Input: part model. Units: mm. Frame: model coordinates. A direction names the side the tool comes from. Coordinates: 2 decimals unless noted, no trailing zeros. Order: outer loops, then holes, each group sorted by start corner. A loop starts at its lowest first (then second) coordinate and runs counter-clockwise, first axis right, second up. Notation, with made-up numbers: (46.5, 18.5) -> (87.5, 18.5) arc R29 ccw to (87.5, 49.5) -> close; hole circle Ø10 at (50, 0.25). An arc over 180 degrees is marked (long way). Write each question's results on one line, items separated by ' | '.
Autodesk Inventor part; units mm, degrees
ref_plane "YZ Plane" through (0, 0, 0) normal (1, 0, 0) x (0, 1, 0)
ref_plane "XZ Plane" through (0, 0, 0) normal (0, 1, 0) x (-1, 0, 0)
ref_plane "XY Plane" through (0, 0, 0) normal (0, 0, 1) x (1, 0, 0)
sketch "Schizzo1" plane through (0, 0, 0) normal (0, 0, 1) x (1, 0, 0)
  circle A0 centre (0, 0) radius 18.5
  dimension "d0" = 37
extrude "Estrusione1" add sketch "Schizzo1" along normal blind 69
sketch "Schizzo2" plane through (0, 0, 0) normal (0, 0, -1) x (-1, 0, 0)
  line L0 (0, 0) -> (15.3, 0)
  line L1 (0, 0) -> (15.3, 0) construction
  point P0 (7.65, 13.2502)
  point P1 (-7.65, 13.2502)
  point P2 (-15.3, 0)
  point P3 (-7.65, -13.2502)
  point P4 (7.65, -13.2502)
  dimension "d3" = 15.3
  dimension "d4" = 0
  dimension "d7" = 360
hole "Foro1" at (7.65, 13.2502, 0) at (-7.65, 13.2502, 0) at (15.3, 0, 0) at (7.65, -13.2502, 0) at (-7.65, -13.2502, 0) at (-15.3, 0, 0) direction (0, 0, 1) diameter 2.459 depth 9 tip angle 118
sketch "Schizzo3" plane through (0, 0, 0) normal (0, 0, -1) x (-1, 0, 0)
  circle A0 centre (0, 0) radius 18.5
  line L0 (0, 18.5) -> (0, -0.9)
  line L1 (0, -0.9) -> (0, -6.9)
  circle A1 centre (0, -6.9) radius 6
  dimension "d16" = 19.4
  dimension "d17" = 6
  dimension "d18" = 12
extrude "Estrusione2" add sketch "Schizzo3" along normal blind 6 contours A1
sketch "Schizzo4" plane through (0, -6.9, -6) normal (0, 0, -1) x (-1, 0, 0)
  circle A0 centre (0, 0) radius 6
  circle A1 centre (0, 0) radius 3
  point P0 (0, 6.9)
  dimension "d21" = 6
extrude "Estrusione3" add sketch "Schizzo4" along normal blind 15 contours A1
sketch "Schizzo5" plane through (0, -6.9, -21) normal (0, 0, -1) x (-1, 0, 0)
  circle A0 centre (0, 0) radius 3
  circle A1 centre (0, 0) radius 3
  line L0 (0, -3) -> (0, 2.5)
  line L1 (0, -3) -> (5.5, -3) construction
  line L2 (22.7528, -2.6034) -> (26.4877, -2.6034) construction
  line L3 (0, 2.5) -> (-1.6583, 2.5)
  line L4 (0, 2.5) -> (1.6583, 2.5)
  point P0 (0, 6.9)
  dimension "d24" = 6
  dimension "d25" = 5.5
  dimension "d26" = 90
extrude "Estrusione4" cut sketch "Schizzo5" against normal blind 12 contours L4 L3 A0
properties part number "29_Motore_6mm"
(1) Pin query (flat end, axial travel): P1, Ø4, axis at x = -7.65, y = 13.25, coming from the -Z side; P2, Ø1, axis at x = 0.5, z = -17.5, coming from the +Y side; P3, Ø10, axis at x = -10.5, z = 29, coming from the +Y side. Return the tip coordinate at first contact, or that it passes through.
Return value:
P1: z = 0 | P2: y = -4.4 | P3: y = 17.66
(2) Cut plane B-B, the plane y = -6.9. Return loops of the section in (x, z), plus the area to 3 significant figures.
Return value:
outline: (-17.17, 0) -> (-6, 0) -> (-6, -6) -> (-3, -6) -> (-3, -21) -> (3, -21) -> (3, -6) -> (6, -6) -> (6, 0) -> (17.17, 0) -> (17.17, 69) -> (-17.17, 69) -> close | area: 2,530 mm2
(3) Mould query, pull axis X, two halves, no side actions, for faces 4 (the face through (-14.552, -0.976, 4.563)), 5 (the face through (-4.01, 18.06, 34.02)), 6 (the face through (3, -8, -6)), 7 (the face through (-7.179, -12.114, 4.563)). Classes: +X half, -X half, draft (parallel to the pull), parting line (faces both ways), or undercut.
Return value:
face 4: undercut | face 5: parting line | face 6: draft | face 7: undercut
(4) Cut plane D-D, the plane z = -12.5. Return loops of the section in (x, y).
Return value:
outline: (-1.66, -4.4) arc R3 ccw (long way) to (1.66, -4.4) -> close
(5) Cut plane A-A, the plane x = 0. Return loops of the section in (y, z).
Return value:
outline: (-18.5, 0) -> (-12.9, 0) -> (-12.9, -6) -> (-9.9, -6) -> (-9.9, -21) -> (-4.4, -21) -> (-4.4, -9) -> (-3.9, -9) -> (-3.9, -6) -> (-0.9, -6) -> (-0.9, 0) -> (18.5, 0) -> (18.5, 69) -> (-18.5, 69) -> close
(6) Line query: line 1 along Y through (x, z) = (7, 2); line 2 along Z through (x, y) = (5, -7.5); line 3 along Y through (x, z) = (12, 36). Output: solid intervals per line, ascending. Write a range as from..to.
Return value:
line 1: -17.12..-14.29, -12.21..12.21, 14.29..17.12 | line 2: -6..69 | line 3: -14.08..14.08
(7) Cut plane C-C, the plane z = 16. Return loops of the section in (x, y), plus the area to 3 significant figures.
Return value:
outline: circle Ø37 at (0, 0) | area: 1,080 mm2
(8) Reachability of faces 1 (the face through (0, -7, -21)), 2 (the face through (4.42, -10.96, -2.96)), 3 (the face through (0, -4.4, -15)) from +Z, -Z, +X, -X, +Y, -Y: full face, straight path, thin tool, end or side. Return the list, or none.
Return value:
face 1: -Z, +X, -X, +Y, -Y | face 2: -Z | face 3: -Z, +X, -X, +Y
